```python
from build123d import *

# Parameters (mm, degrees)
SKETCH1_W           = 27
SKETCH1_H           = 23
BOSS_EXTRUDE1_DEPTH = 2
SKETCH2_W           = 21
SKETCH2_H           = 14
BOSS_EXTRUDE2_DEPTH = 2
SKETCH3_W           = 21
SKETCH3_H           = 6
CUT_EXTRUDE1_DEPTH  = 2


with BuildPart() as part:
    # Sketch1 → Boss-Extrude1 (new body)
    with BuildSketch(Plane.XY):
        Rectangle(SKETCH1_W, SKETCH1_H)
    extrude(amount=BOSS_EXTRUDE1_DEPTH)

    # Sketch2 → Boss-Extrude2 (add)
    with BuildSketch(Plane.XY.offset(2)):
        with Locations((0, 1.5)):
            Rectangle(SKETCH2_W, SKETCH2_H)
    extrude(amount=BOSS_EXTRUDE2_DEPTH)

    # Sketch3 → Cut-Extrude1 (cut)
    with BuildSketch(Plane.XY.offset(2)):
        with Locations((0, -8.5)):
            Rectangle(SKETCH3_W, SKETCH3_H)
    extrude(amount=-CUT_EXTRUDE1_DEPTH, mode=Mode.SUBTRACT)


solid = part.part
```
Part model, mm, in its own coordinate system. A direction names the side the tool comes from. Coordinates: 2 decimals unless noted, no trailing zeros. Order: outer loops, then holes, each group sorted by start corner. A loop starts at its lowest first (then second) coordinate and runs counter-clockwise, first axis right, second up. Notation, with made-up numbers: (66, 63) -> (91, 63) arc R31 ccw to (91, 92) -> close; hole circle Ø2 at (49, 29). An arc over 180 degrees is marked (long way). Put each result on its own line as item: value. Start each with the question number.
(1) Band-saw the part on B-B (z = 0.55). Give the cut face in (x, y), then the cut area to 3 significant figures.
(2) Which spindle directions (+Z, -Z, +X, -X, +Y, -Y) get a long thin tool onto all of the face, cutting with end or side? Do faces 1 (the face through (0, 3, 0)), 2 (the face through (10.5, 1, 3)), 3 (the face through (-10.5, 1, 3)), 4 (the face through (0, 8.5, 3)), 5 (the face through (0, -5.5, 2)). Say none if no direction does.
(3) Band-saw the part on A-A (y = -7.5). Give the cut face in (x, z), then the cut area to 3 significant figures.
(4) Band-saw the part on C-C (x = 8.5). Give the cut face in (y, z), then the cut area to 3 significant figures.
(5) Band-saw the part on D-D (y = -4.5). Give the cut face in (x, z), then the cut area to 3 significant figures.
(6) Probe line 1 along X through (y, z) = (-6.25, 1.2); line 2 along Y through (x, z) = (8.75, 3.2); line 3 along Y through (x, z) = (-6.25, 1.8). List the from-to ranges inside material, lowest first. Write a range as [from, to].
(7) Pin check, flat tips, straight feed: pin 1 Ø5 at (x, y) = (-0.5, -8.5) entering from -Z; pin 2 Ø0.6 at (y, z) = (-2, 2.5) entering from +X; pin 3 Ø1 at (y, z) = (2, 3.5) entering from -X. Stop position of each tip, or through.
(8) Mould opens along X. For faces 6 (the face through (10.5, -9, 1)), 7 (the face through (0, 9, 2)), 8 (the face through (-10.5, -9, 1)), 9 (the face through (-13.5, 0, 1)) say: pulls with the +X half, pulls with the -X half, needs draft (parallel to the pull), parting line crosses it, or undercut.
Determined:
1. outline: (-13.5, -11.5) -> (-10.5, -11.5) -> (-10.5, -5.5) -> (10.5, -5.5) -> (10.5, -11.5) -> (13.5, -11.5) -> (13.5, 11.5) -> (-13.5, 11.5) -> close
1. area: 495 mm²
2. face 1: -Z, +X, -X, +Y, -Y
2. face 2: +Z, +X, +Y, -Y
2. face 3: +Z, -X, +Y, -Y
2. face 4: +Z, +X, -X, +Y
2. face 5: +Z, -Z, -Y
3. outline: (-13.5, 0) -> (-10.5, 0) -> (-10.5, 2) -> (-13.5, 2) -> close; (10.5, 0) -> (13.5, 0) -> (13.5, 2) -> (10.5, 2) -> close
3. area: 12.0 mm²
4. outline: (-5.5, 0) -> (11.5, 0) -> (11.5, 2) -> (8.5, 2) -> (8.5, 4) -> (-5.5, 4) -> close
4. area: 62.0 mm²
5. outline: (-13.5, 0) -> (13.5, 0) -> (13.5, 2) -> (10.5, 2) -> (10.5, 4) -> (-10.5, 4) -> (-10.5, 2) -> (-13.5, 2) -> close
5. area: 96.0 mm²
6. line 1: x = [-13.5, -10.5], [10.5, 13.5]
6. line 2: y = [-5.5, 8.5]
6. line 3: y = [-5.5, 11.5]
7. pin 1: passes through
7. pin 2: stops at x = 10.5
7. pin 3: stops at x = -10.5
8. face 6: undercut
8. face 7: needs draft
8. face 8: undercut
8. face 9: pulls with the -X half
